```python
from build123d import *

# Parameters (mm, degrees)
F0_W     = 127
F0_H     = 304.8
F0_W_2   = 101.6
F0_H_2   = 152.4
F0_W_3   = 76.2
F0_H_3   = 121.92
F0_W_4   = 50.8
F0_H_4   = 114.3
F1_DEPTH = 50.8
F2_DEPTH = 5
F3_DEPTH = 38.1
F4_R     = 10


with BuildPart() as f1:
    # F0 (on Front) → F1 (new body)
    with BuildSketch(Plane.XZ):
        with Locations((0, -38.1)):
            Rectangle(F0_W, F0_H)
        Rectangle(F0_W_2, F0_H_2, mode=Mode.SUBTRACT)
        Rectangle(F0_W_2, F0_H_2)
        Rectangle(F0_W_3, F0_H_3, mode=Mode.SUBTRACT)
        Rectangle(F0_W_3, F0_H_3)
        Rectangle(F0_W_4, F0_H_4, mode=Mode.SUBTRACT)
    extrude(amount=-F1_DEPTH)

    # F0 (on Front) → F2 (cut)
    with BuildSketch(Plane.XZ):
        Rectangle(F0_W_2, F0_H_2)
        Rectangle(F0_W_3, F0_H_3, mode=Mode.SUBTRACT)
    extrude(amount=-F2_DEPTH, mode=Mode.SUBTRACT)

    # F0 (on Front) → F3 (cut)
    with BuildSketch(Plane.XZ):
        Rectangle(F0_W_3, F0_H_3)
        Rectangle(F0_W_4, F0_H_4, mode=Mode.SUBTRACT)
    extrude(amount=-F3_DEPTH, mode=Mode.SUBTRACT)

    # F4
    f4_edges = [f1.edges().sort_by_distance(p)[0] for p in [
        (-25.4, 44.45, 57.15),
        (25.4, 44.45, 57.15),
        (-25.4, 44.45, -57.15),
        (25.4, 44.45, -57.15),
    ]]
    fillet(f4_edges, radius=F4_R)


solid = f1.part
```
Source: CAD feature listing. Evaluate the final solid. Frame: model axes, mm. A direction names the side the tool comes from. Round coordinates to 2 decimals unless told otherwise and drop trailing zeros. Loops run counter-clockwise (first coordinate to the right, second up) from the corner with the lowest first, then second, coordinate; pieces in that order, holes last. Notation, with made-up numbers: M 55.5,27.5 L 77.5,27.5 A14 ccw 77.5,46.5 Z; hole C 31,4.5 d11. An arc over 180 degrees is marked long. Use a Markdown table: item, result. Add a question column.
1. Set-up query: faces 5 (the flat face through (-1, 0, -104)), 6 (the flat face through (44, 5, 1)), 7 (the cylindrical face through (22.55, 44.54, 54.14)). Return all of +Z, -Z, +X, -X, +Y, -Y with unobstructed straight access to the full face (end or side cutting, diameter ignored); none if empty.
2. Contact query for flat-ended pins moving along their axis: pin 1 (4 mm diameter, centred on x = -44, z = -141, fed in from -Y); pin 2 (2 mm diameter, centred on x = 6.5, z = 55.5, fed in from +Y). Output: stop coordinate, or through.
3. Cut plane B-B, the plane y = 8.5. Output: boundary loops of the cut face in (x, z), and give its area (3 significant figures).
4. Cut plane D-D, the plane x = -32.5. Output: boundary loops of the cut face in (y, z).
5. Cut plane C-C, the plane z = 27.5. Output: boundary loops of the cut face in (x, y).
6. Cut plane A-A, the plane x = -2.5. Output: boundary loops of the cut face in (y, z), and give its area (3 significant figures).
7. Ray query, line 1 along X through (y, z) = (17, -13.5); line 2 along Z through (x, y) = (8, 21); line 3 along Z through (x, y) = (-48.5, 2). Return the intervals inside material, ascending. Write a range as [from, to].
8. Pull-direction query (Z, two-part tool) for faces 1 (the flat face through (-1, 21, 60.96)), 2 (the flat face through (-1, 25, -190.5)), 3 (the flat face through (63.5, 25, -40)), 4 (the cylindrical face through (22.39, 44.54, -54.3)); classes: +Z half, -Z half, draft (parallel to the pull), parting line (faces both ways), or undercut.
Solution:
| question | item | result |
|---|---|---|
| 1 | face 5 | +Z, -Z, +X, -X, -Y |
| 1 | face 6 | -Y |
| 1 | face 7 | +Y, -Y |
| 2 | pin 1 | stops at y = 0 |
| 2 | pin 2 | passes through |
| 3 | outline | M -63.5,-190.5 L 63.5,-190.5 L 63.5,114.3 L -63.5,114.3 Z; hole M -38.1,-60.96 L 38.1,-60.96 L 38.1,60.96 L -38.1,60.96 Z |
| 3 | area | 29,400 mm2 |
| 4 | outline | M 0,-190.5 L 50.8,-190.5 L 50.8,114.3 L 0,114.3 L 0,76.2 L 5,76.2 L 5,60.96 L 38.1,60.96 L 38.1,-60.96 L 5,-60.96 L 5,-76.2 L 0,-76.2 Z |
| 5 | outline | M -63.5,0 L -50.8,0 L -50.8,5 L -38.1,5 L -38.1,38.1 L -25.4,38.1 L -25.4,50.8 L -63.5,50.8 Z; M 25.4,38.1 L 38.1,38.1 L 38.1,5 L 50.8,5 L 50.8,0 L 63.5,0 L 63.5,50.8 L 25.4,50.8 Z |
| 6 | outline | M 0,-190.5 L 50.8,-190.5 L 50.8,-57.15 L 38.1,-57.15 L 38.1,-60.96 L 5,-60.96 L 5,-76.2 L 0,-76.2 Z; M 0,76.2 L 5,76.2 L 5,60.96 L 38.1,60.96 L 38.1,57.15 L 50.8,57.15 L 50.8,114.3 L 0,114.3 Z |
| 6 | area | 9,230 mm2 |
| 7 | line 1 | x = [-63.5, -38.1], [38.1, 63.5] |
| 7 | line 2 | z = [-190.5, -60.96], [60.96, 114.3] |
| 7 | line 3 | z = [-190.5, -76.2], [76.2, 114.3] |
| 8 | face 1 | undercut |
| 8 | face 2 | -Z half |
| 8 | face 3 | draft |
| 8 | face 4 | undercut |
